Here's how the part is built. I have some questions about the finished solid (model axes, mm). A direction names the side the tool comes from. Round coordinates to 2 decimals unless told otherwise and drop trailing zeros. Loops run counter-clockwise (first coordinate to the right, second up) from the corner with the lowest first, then second, coordinate; pieces in that order, holes last. Notation, with made-up numbers: (2, 76.25) -> (6, 76.25) arc R23 ccw to (6, 92.25) -> close; hole circle Ø4 at (32.5, 3). An arc over 180 degrees is marked (long way). Use CSV: the item, a comma, the result in double quotes. Start each with the question number.
from build123d import *

# Parameters (mm, degrees)
F0_R     = 20
F1_DEPTH = 5
F5_T     = -2.5


# Not quite as in the source:
# - a fillet or chamfer that OpenCascade refuses, or shapes differently, is made with other operations: its cross-section is extruded or revolved along the edge and cut away or added


with BuildPart() as f1:
    # F0 (on Top) → F1 (new body)
    with BuildSketch(Plane.XY):
        Circle(F0_R)
    extrude(amount=F1_DEPTH)

    # F2 (on Right) → F3 (revolve)
    with BuildSketch(Plane.YZ):
        with BuildLine():
            Line((0, 0.953980596), (0, 47.7081678201))
            ThreePointArc((0, 47.7081678201), (-23.377093612, 24.331074208), (0, 0.953980596))
        make_face()
    revolve(axis=Axis((0, 0, 23.85408391), (0, 0, 1)))

    # F4: fillet of radius 5 on 1 edges, made by hand

    # F4_s1 → F4_t2 (revolve)
    with BuildSketch(Plane.YZ):
        with BuildLine():
            ThreePointArc((-20, 5), (-18.5807849657, 8.0440971034), (-19.4078057687, 11.2993597778))
            Line((-19.4078057687, 11.2993597778), (-19.3247851585, 11.3551054348))
            ThreePointArc((-19.3247851585, 11.3551054348), (-16.5075665861, 7.9200007382), (-13.0890367821, 5.0826923763))
            Line((-13.0890367821, 5.0826923763), (-13.1452681871, 4.9))
            ThreePointArc((-13.1452681871, 4.9), (-16.5726340935, 4.9), (-19.9288232744, 4.9297584615))
            Line((-19.9288232744, 4.9297584615), (-20, 5))
        make_face()
    revolve(axis=Axis((0, 0, 5), (0, 0, -1)))

    # F5
    f5_openings = [f1.faces().sort_by_distance(p)[0] for p in [
        (0, 0, 0),
    ]]
    offset(amount=F5_T, openings=f5_openings)


solid = f1.part
Q1. Will these pins go through, and if not, where does the flat tip stop? pin 1 Ø5 at (x, y) = (-6.5, 4) entering from +Z; pin 2 Ø2 at (x, y) = (16.5, -2.5) entering from +Z; pin 3 Ø1.5 at (x, z) = (-14, 36.5) entering from +Y.
Q2. I need wall thicknesses on line 1 along X through (y, z) = (0, 2.1); line 2 along Z through (x, y) = (16, -11). Which ranges of each line are inside material? Lowest first, please.
Q3. For faces 1 (the flat face through (0, -18, 0)), 2 (the cylindrical face through (-4.336, -19.524, 2.465)), which set-ups out of +Z, -Z, +X, -X, +Y, -Y let a thin tool reach every point of the face, with its end or its side?
Q4. I want a section at D-D, the plane z = 23.5. List the corners of the cut face in (x, y) for me.
Q5. I want a section at C-C, the plane z = 8. List the corners of the cut face in (x, y) for me.
Q6. I want a section at A-A, the plane x = 0. List the corners of the cut face in (y, z) for me.
Values found:
1,pin 1,"z = 47.14"
1,pin 2,"z = 41.66"
1,pin 3,"y = 15.15"
2,line 1,"-20 to -17.5, 17.5 to 20"
2,line 2,"0 to 5.71, 11.31 to 16.66, 32 to 37.35"
3,face 1,"-Z, +X, -X, +Y, -Y"
3,face 2,"-Z"
4,outline,"circle Ø46.72 at (0, 0); hole circle Ø41.72 at (0, 0)"
5,outline,"circle Ø37.17 at (0, 0); hole circle Ø32.15 at (0, 0)"
6,outline,"(-20, 0) -> (-17.5, 0) -> (-17.5, 4.09) arc R7.5 ccw to (-17.33, 12.69) arc R20.88 cw (long way) to (17.33, 12.69) arc R7.5 ccw to (17.5, 4.09) -> (17.5, 0) -> (20, 0) -> (20, 5) arc R5 cw to (19.41, 11.3) arc R23.38 ccw (long way) to (-19.41, 11.3) arc R5 cw to (-20, 5) -> close"
